Check sheet for the modelled part. Datum: model origin and axes. Units: mm. Face numbers are marked on the shaded views. A direction names the side the tool comes from. Round coordinates to 2 decimals unless told otherwise and drop trailing zeros. Write each loop counter-clockwise with the first axis right and the second up, starting at its lowest first coordinate (ties: lowest second). Pieces come first, ordered by that corner, then holes.
Item 1: Section check C-C, the plane x = -87.5. Record the cut outline in (y, z).
Item 2: Depth check by flat-ended pin: pin 1 (12 mm diameter, centred on x = -23.5, y = 7.5, fed in from +Z); pin 2 (3.5 mm diameter, centred on x = -33.14, z = 14.18, fed in from +Y); pin 3 (4.5 mm diameter, centred on y = 8, z = 4, fed in from -X). Enter the tip coordinate at first touch or a pass-through.
Item 3: Section check D-D, the plane z = 22. Record the cut outline in (x, y), plus the area to 3 significant figures.
Item 4: Section check A-A, the plane z = -18.5. Record the cut outline in (x, y).
Item 5: Material ranges on line 1 along Z through (x, y) = (27.5, 25.25); line 2 along X through (y, z) = (14.5, 22.5); line 3 along Y through (x, z) = (-109.5, 27.5), recorded low to high.
Item 6: Section check B-B, the plane y = 5.75. Record the cut outline in (x, z), plus the area to 3 significant figures.
Item 7: Set-up check for the marked faces 1, 2 and 3: record each of +Z, -Z, +X, -X, +Y, -Y from which the full face is reachable in a straight line by a thin tool's end or side.
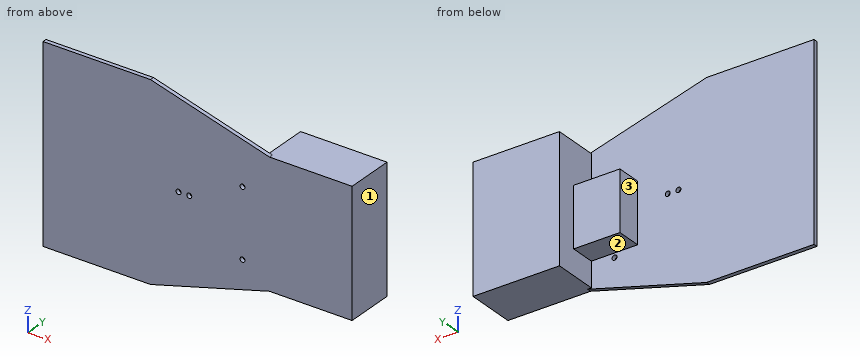
from build123d import *

# Parameters (mm, degrees)
SKETCH1_W           = 65
SKETCH1_H           = 116
SKETCH1_W_2         = 50
SKETCH1_H_2         = 76
BOSS_EXTRUDE1_DEPTH = 2.5
SKETCH2_R           = 1.5
CUT_EXTRUDE1_DEPTH  = 142.460566572
SKETCH3_R           = 1.5
CUT_EXTRUDE2_DEPTH  = 142.460566572
SKETCH4_W           = 28
SKETCH4_H           = 36
BOSS_EXTRUDE2_DEPTH = 15
SKETCH5_W           = 52.3
SKETCH5_H           = 76
BOSS_EXTRUDE3_DEPTH = 27


with BuildPart() as part:
    # Sketch1 → Boss-Extrude1 (new body)
    with BuildSketch(Plane(origin=(0, 0, 0), x_dir=(1, 0, 0), z_dir=(0, 1, 0))):
        with Locations((-89.136826853, -14.17564858)):
            Rectangle(SKETCH1_W, SKETCH1_H)
        Polygon((15.363173147, -14.17564858), (-56.636826853, -14.17564858), (-56.636826853, -72.17564858), (15.363173147, -52.17564858), align=None)
        Polygon((15.363173147, 23.82435142), (-56.636826853, 43.82435142), (-56.636826853, -14.17564858), (15.363173147, -14.17564858), align=None)
        with Locations((40.363173147, -14.17564858)):
            Rectangle(SKETCH1_W_2, SKETCH1_H_2)
    extrude(amount=BOSS_EXTRUDE1_DEPTH)

    # Sketch2 → Cut-Extrude1 (cut, through all)
    with BuildSketch(Plane(origin=(0, 2.5, 0), x_dir=(1, 0, 0), z_dir=(0, 1, 0))):
        with Locations(Location((-39.636826853, -14.17564858, 0), (0, 0, 270))):
            Circle(SKETCH2_R)
        with Locations(Location((-33.136826853, -14.17564858, 0), (0, 0, 270))):
            Circle(SKETCH2_R)
    extrude(amount=-CUT_EXTRUDE1_DEPTH, mode=Mode.SUBTRACT)

    # Sketch3 → Cut-Extrude2 (cut, through all)
    with BuildSketch(Plane(origin=(0, 2.5, 0), x_dir=(1, 0, 0), z_dir=(0, 1, 0))):
        with Locations(Location((-0.936826853, 11.352129198, 0), (0, 0, 270))):
            Circle(SKETCH3_R)
        with Locations(Location((-0.936826853, -29.947870802, 0), (0, 0, 270))):
            Circle(SKETCH3_R)
    extrude(amount=-CUT_EXTRUDE2_DEPTH, mode=Mode.SUBTRACT)

    # Sketch4 → Boss-Extrude2 (add)
    with BuildSketch(Plane(origin=(0, 2.5, 0), x_dir=(1, 0, 0), z_dir=(0, 1, 0))):
        with Locations((-0.936826853, -9.297870802)):
            Rectangle(SKETCH4_W, SKETCH4_H)
    extrude(amount=BOSS_EXTRUDE2_DEPTH)

    # Sketch5 → Boss-Extrude3 (add)
    with BuildSketch(Plane(origin=(0, 2.5, 0), x_dir=(1, 0, 0), z_dir=(0, 1, 0))):
        with Locations((39.213173147, -14.17564858)):
            Rectangle(SKETCH5_W, SKETCH5_H)
    extrude(amount=BOSS_EXTRUDE3_DEPTH)


solid = part.part
Values found:
1. outline: (0, -43.82) - (2.5, -43.82) - (2.5, 72.18) - (0, 72.18) - close
2. pin 1: stops at z = 63.89
2. pin 2: stops at y = 2.5
2. pin 3: stops at x = -14.94
3. outline: (-121.64, 0) - (65.36, 0) - (65.36, 29.5) - (13.06, 29.5) - (13.06, 17.5) - (-14.94, 17.5) - (-14.94, 2.5) - (-121.64, 2.5) - close
3. area: 2,300 mm2
4. outline: (-121.64, 0) - (65.36, 0) - (65.36, 29.5) - (13.06, 29.5) - (13.06, 2.5) - (-121.64, 2.5) - close
5. line 1: z = -23.82 to 52.18
5. line 2: x = -14.94 to 65.36
5. line 3: y = 0 to 2.5
6. outline: (-14.94, -8.7) - (13.06, -8.7) - (13.06, -23.82) - (65.36, -23.82) - (65.36, 52.18) - (13.06, 52.18) - (13.06, 27.3) - (-14.94, 27.3) - close
6. area: 4,980 mm2
7. face 1: +Z, -Z, +X, +Y, -Y
7. face 2: -Z, -X, +Y
7. face 3: +Z, -Z, -X, +Y
